Build history of the part. All positions in model axes, mm. Coordinates: 2 decimals unless noted, no trailing zeros. Loops run counter-clockwise (first coordinate to the right, second up) from the corner with the lowest first, then second, coordinate; pieces in that order, holes last.
(1) Slice it at A-A (z = 2.7). Give the number of separate pieces and of enclosed holes in the cut face, and give its area (3 significant figures).
(2) Flat gauge pins, fed straight in: P1, Ø3, axis at x = -20.1, y = -12, coming from the +Z side; P2, Ø12, axis at x = 15.5, y = -5, coming from the -Z side. Where does each tip first touch, or does it go through?
(3) Slice it at D-D (x = 0). Give the cut face in (y, z).
(4) Wall check: L1, parallel to Y at x = -20, z = 3.9; L2, parallel to X at y = -23, z = 3.95; L3, parallel to X at y = 36, z = 3.6. Give the ranges that are in metal, low to high.
(5) Slice it at B-B (y = -22). Give the cut face in (x, z), and give its area (3 significant figures).
(6) Slice it at C-C (x = 25). Give the cut face in (y, z).
from build123d import *

# Parameters (mm, degrees)
SKETCH_1_W          = 60
SKETCH_1_H          = 120
SKETCH_1_R          = 1.6
SKETCH_1_R_2        = 2.15
EXTRUDE_3_DEPTH     = 6
SKETCH_9_R          = 1.6
CUT_EXTRUDE_1_DEPTH = 6
FILLET_1_R          = 10
SKETCH_10_R         = 1.6
CUT_EXTRUDE_2_DEPTH = 10
SKETCH_11_R         = 15
CUT_EXTRUDE_3_DEPTH = 10
EXTRUDE_START       = -6
SKETCH_12_R         = 1.6
EXTRUDE_4_DEPTH     = 6
EXTRUDE_5_DEPTH     = 6
SKETCH_14_R         = 15
CUT_EXTRUDE_4_DEPTH = 68.349832962


with BuildPart() as part:
    # 草图1 → 凸台-拉伸3 (new body)
    with BuildSketch(Plane.XY):
        Rectangle(SKETCH_1_W, SKETCH_1_H)
        with Locations((0, 50.5)):
            Circle(SKETCH_1_R, mode=Mode.SUBTRACT)
        with Locations((20, -50)):
            Circle(SKETCH_1_R_2, mode=Mode.SUBTRACT)
        with Locations((-20, -50)):
            Circle(SKETCH_1_R_2, mode=Mode.SUBTRACT)
        with Locations((13.423393759, 42.75)):
            Circle(SKETCH_1_R, mode=Mode.SUBTRACT)
        with Locations((13.423393759, 27.25)):
            Circle(SKETCH_1_R, mode=Mode.SUBTRACT)
        with Locations((0, 19.5)):
            Circle(SKETCH_1_R, mode=Mode.SUBTRACT)
        with Locations((-13.423393759, 27.25)):
            Circle(SKETCH_1_R, mode=Mode.SUBTRACT)
        with Locations((-13.423393759, 42.75)):
            Circle(SKETCH_1_R, mode=Mode.SUBTRACT)
        with BuildLine():
            Line((6, 42), (6, 28))
            ThreePointArc((6, 28), (0, 22), (-6, 28))
            Line((-6, 28), (-6, 42))
            ThreePointArc((-6, 42), (0, 48), (6, 42))
        make_face(mode=Mode.SUBTRACT)
    extrude(amount=EXTRUDE_3_DEPTH)

    # 草图9 → 切除-拉伸1 (cut)
    with BuildSketch(Plane.XY.offset(6)):
        with Locations((20.1, -22)):
            Circle(SKETCH_9_R)
        with Locations((20.1, -2)):
            Circle(SKETCH_9_R)
        with Locations((20.1, -12)):
            Circle(SKETCH_9_R)
        with Locations((-20.1, -2)):
            Circle(SKETCH_9_R)
        with Locations((-20.1, -12)):
            Circle(SKETCH_9_R)
        with Locations((-20.1, -22)):
            Circle(SKETCH_9_R)
    extrude(amount=-CUT_EXTRUDE_1_DEPTH, mode=Mode.SUBTRACT)

    # 圆角1
    fillet_1_edges = [part.edges().sort_by_distance(p)[0] for p in [
        (30, -60, 3),
        (-30, -60, 3),
        (-30, 60, 3),
        (30, 60, 3),
    ]]
    fillet(fillet_1_edges, radius=FILLET_1_R)

    # 草图10 → 切除-拉伸2 (cut)
    with BuildSketch(Plane(origin=(0, 0, 0), x_dir=(-1, 0, 0), z_dir=(0, 0, -1))):
        with Locations((-20, 50)):
            Circle(SKETCH_10_R)
        with Locations((-25, 10)):
            Circle(SKETCH_10_R)
        with Locations((25, 10)):
            Circle(SKETCH_10_R)
        with Locations((20, 50)):
            Circle(SKETCH_10_R)
    extrude(amount=-CUT_EXTRUDE_2_DEPTH, mode=Mode.SUBTRACT)

    # 草图11 → 切除-拉伸3 (cut)
    with BuildSketch(Plane.XY.offset(6)):
        with Locations((0, 28)):
            Circle(SKETCH_11_R)
    extrude(amount=-CUT_EXTRUDE_3_DEPTH, mode=Mode.SUBTRACT)

    # 草图12 → 凸台-拉伸4 (add)
    with BuildSketch(Plane.XY.offset(6).offset(EXTRUDE_START)):
        with BuildLine():
            ThreePointArc((5.994789404, 41.75), (5.99869721, 41.874972853), (6, 42))
            ThreePointArc((6, 42), (0, 48), (-6, 42))
            ThreePointArc((-6, 42), (-5.99869721, 41.874972853), (-5.994789404, 41.75))
            ThreePointArc((-5.994789404, 41.75), (0, 43), (5.994789404, 41.75))
        make_face()
        with Locations((-13.423393759, 42.75)):
            Circle(SKETCH_12_R)
        with Locations((0, 50.5)):
            Circle(SKETCH_12_R)
        with Locations((13.423393759, 42.75)):
            Circle(SKETCH_12_R)
    extrude(amount=EXTRUDE_4_DEPTH)

    # 草图13 → 凸台-拉伸5 (add)
    with BuildSketch(Plane(origin=(0, 0, 0), x_dir=(-1, 0, 0), z_dir=(0, 0, -1)).offset(EXTRUDE_START)):
        with BuildLine():
            ThreePointArc((13.266499161, 35), (0, 27), (-13.266499161, 35))
            ThreePointArc((-13.266499161, 35), (-14.611734824, 31.390752932), (-14.993484161, 27.557922277))
            ThreePointArc((-14.993484161, 27.557922277), (-14.976641564, 27.163215996), (-14.949410055, 26.769090172))
            ThreePointArc((-14.949410055, 26.769090172), (0, 13), (14.949410055, 26.769090172))
            ThreePointArc((14.949410055, 26.769090172), (14.976641564, 27.163215996), (14.993484161, 27.557922277))
            ThreePointArc((14.993484161, 27.557922277), (14.998370952, 27.77893713), (15, 28))
            ThreePointArc((15, 28), (14.560176637, 31.605725487), (13.266499161, 35))
        make_face()
    extrude(amount=EXTRUDE_5_DEPTH)

    # 草图14 → 切除-拉伸4 (cut, through all)
    with BuildSketch(Plane(origin=(0, 0, 0), x_dir=(-1, 0, 0), z_dir=(0, 0, -1))):
        with Locations((0, 42)):
            Circle(SKETCH_14_R)
    extrude(amount=-CUT_EXTRUDE_4_DEPTH, mode=Mode.SUBTRACT)


solid = part.part
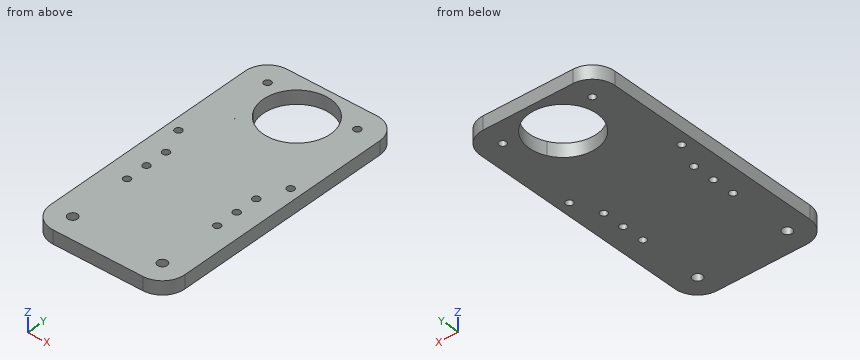
Response values:
1. separate pieces: 1
1. enclosed holes: 15
1. area: 6,300 mm2
2. P1: passes through
2. P2: stops at z = 0
3. outline: (-60, 0) - (27, 0) - (27, 6) - (-60, 6) - close; (57, 0) - (60, 0) - (60, 6) - (57, 6) - close
4. L1: y = -60 to -52.15, -47.85 to -23.6, -20.4 to -13.6, -10.4 to -3.6, -0.4 to 48.4, 51.6 to 60
4. L2: x = -30 to -21.35, -18.85 to 18.85, 21.35 to 30
4. L3: x = -30 to -13.75, 13.75 to 30
5. outline: (-30, 0) - (-21.7, 0) - (-21.7, 6) - (-30, 6) - close; (-18.5, 0) - (18.5, 0) - (18.5, 6) - (-18.5, 6) - close; (21.7, 0) - (30, 0) - (30, 6) - (21.7, 6) - close
5. area: 322 mm2
6. outline: (-58.66, 0) - (8.4, 0) - (8.4, 6) - (-58.66, 6) - close; (11.6, 0) - (58.66, 0) - (58.66, 6) - (11.6, 6) - close
